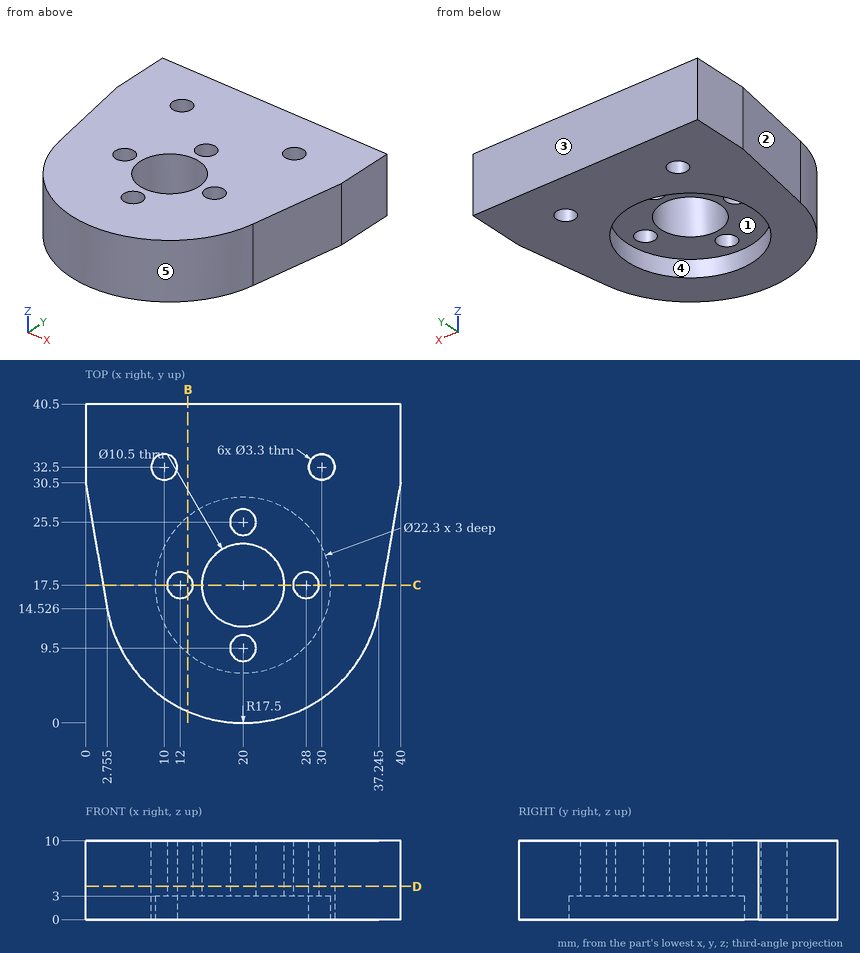
Job drawing, mm, ordinate dimensions from the low corner. One solid piece. A direction names the side the tool comes from. Round coordinates to 2 decimals unless told otherwise and drop trailing zeros. Loops run counter-clockwise (first coordinate to the right, second up) from the corner with the lowest first, then second, coordinate; pieces in that order, holes last. Notation, with made-up numbers: (28, 33) -> (61, 33) arc R27 cw to (61, 72) -> close; hole circle Ø3 at (74.5, 9). An arc over 180 degrees is marked (long way). One line per item, written item: value. Start each with the question number.
Q1. Cut at C-C on y = 17.5. List the corners of the cut face in (x, z).
Q2. Cut at D-D on z = 4.25. Count the separate pieces of the cut face and the enclosed holes in it, plus the area to 3 significant figures.
Q3. Drop flat-ended pins along their axis: pin 1 Ø8 at (x, y) = (29.5, 18) entering from -Z; pin 2 Ø3 at (x, y) = (28, 17.5) entering from -Z; pin 3 Ø1.5 at (y, z) = (26, 2.5) entering from +X; pin 4 Ø3 at (y, z) = (6, 4) entering from -X. Give the stop position or say it passes through.
Q4. Probe line 1 along Y through (x, z) = (29, 2.5) (1 decimal); line 2 along Z through (x, y) = (26, 24); line 3 along Y through (x, z) = (11, 7) (1 decimal). List the from-to ranges inside material, lowest first.
Q5. Two-plate mould, pull along X, no slides. Class the marked faces 3, 4 and 5: released by +X, released by -X, zero draft, split by the parting line, or undercut.
Q6. 3-axis set-ups, long thin cutter, end or side, ignore diameter. For the marked faces 1 and 2: which of +Z, -Z, +X, -X, +Y, -Y reach the whole face in a straight line?
Q7. Cut at B-B on x = 13. List the corners of the cut face in (y, z).
Computed:
1. outline: (2.24, 0) -> (8.85, 0) -> (8.85, 3) -> (10.35, 3) -> (10.35, 10) -> (2.24, 10) -> close; (13.65, 3) -> (14.75, 3) -> (14.75, 10) -> (13.65, 10) -> close; (25.25, 3) -> (26.35, 3) -> (26.35, 10) -> (25.25, 10) -> close; (29.65, 3) -> (31.15, 3) -> (31.15, 0) -> (37.76, 0) -> (37.76, 10) -> (29.65, 10) -> close
2. separate pieces: 1
2. enclosed holes: 7
2. area: 1,230 mm²
3. pin 1: z = 0
3. pin 2: through
3. pin 3: x = 39.35
3. pin 4: x = 5.64
4. line 1: 2.5 to 10.9, 24.1 to 31.2, 33.8 to 40.5
4. line 2: 3 to 10
4. line 3: 2.5 to 16.2, 18.8 to 31.2, 33.8 to 40.5
5. face 3: zero draft
5. face 4: undercut
5. face 5: split by the parting line
6. face 1: -Z
6. face 2: +Z, -Z, -X, -Y
7. outline: (1.46, 0) -> (8.82, 0) -> (8.82, 3) -> (16.19, 3) -> (16.19, 10) -> (1.46, 10) -> close; (18.81, 3) -> (26.18, 3) -> (26.18, 0) -> (40.5, 0) -> (40.5, 10) -> (18.81, 10) -> close
